For this review, take the finished solid that the model builds, in its own axes (mm). Face numbers are marked on the shaded views. Round coordinates to 2 decimals unless told otherwise and drop trailing zeros. Order: outer loops, then holes, each group sorted by start corner. A loop starts at its lowest first (then second) coordinate and runs counter-clockwise, first axis right, second up. Notation, with made-up numbers: M 0.5,-0.5 L 37.5,-0.5 A31 ccw 37.5,31.5 Z; hole C 67.25,-22 d7. An arc over 180 degrees is marked long. Use a Markdown table: item, result.
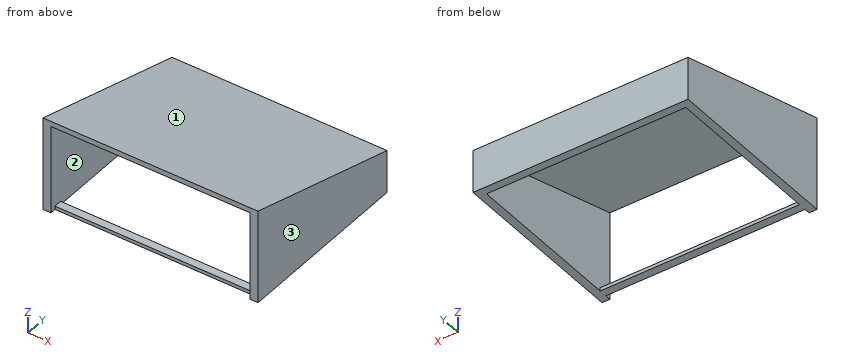
from build123d import *

# Parameters (mm, degrees)
SLOPED_COVER_BLANK_DEPTH                      = 95
SLOPED_COVER_BLANK_DEPTH_BACK                 = 95
OPEN_BOTTOM_AND_FRONT_COVER_CAVITY_DEPTH      = 88
OPEN_BOTTOM_AND_FRONT_COVER_CAVITY_DEPTH_BACK = 88
FRONT_GASKET_COMPRESSION_RAIL_DEPTH           = 95
FRONT_GASKET_COMPRESSION_RAIL_DEPTH_BACK      = 95
FRONT_GASKET_COMPRESSION_RAIL_PROFILE_W       = 3
FRONT_GASKET_COMPRESSION_RAIL_PROFILE_H       = 7


with BuildPart() as part:
    # Sloped Cover Outer Side Profile → Sloped Cover Blank (new, two sides: drawn at the far end of the back side and taken through both)
    with BuildSketch(Plane(origin=(0, 0, 0), x_dir=(0, 0, -1), z_dir=(1, 0, 0)).offset(-SLOPED_COVER_BLANK_DEPTH_BACK)):
        Polygon((-22, 40), (-22, 200), (-60, 200), (-105, 40), align=None)
    extrude(amount=SLOPED_COVER_BLANK_DEPTH + SLOPED_COVER_BLANK_DEPTH_BACK)

    # Open Bottom Cover Cavity Profile → Open Bottom and Front Cover Cavity (cut, two sides: drawn at the far end of the back side and taken through both)
    with BuildSketch(Plane(origin=(0, 0, 0), x_dir=(0, 0, -1), z_dir=(1, 0, 0)).offset(-OPEN_BOTTOM_AND_FRONT_COVER_CAVITY_DEPTH_BACK)):
        Polygon((-18, 38), (-18, 193), (-56, 193), (-101, 38), align=None)
    extrude(amount=OPEN_BOTTOM_AND_FRONT_COVER_CAVITY_DEPTH + OPEN_BOTTOM_AND_FRONT_COVER_CAVITY_DEPTH_BACK, mode=Mode.SUBTRACT)

    # Front Gasket Compression Rail Profile → Front Gasket Compression Rail (add, two sides: drawn at the far end of the back side and taken through both)
    with BuildSketch(Plane(origin=(0, 0, 0), x_dir=(0, 0, -1), z_dir=(1, 0, 0)).offset(-FRONT_GASKET_COMPRESSION_RAIL_DEPTH_BACK)):
        with Locations((-23.5, 48.5)):
            Rectangle(FRONT_GASKET_COMPRESSION_RAIL_PROFILE_W, FRONT_GASKET_COMPRESSION_RAIL_PROFILE_H)
    extrude(amount=FRONT_GASKET_COMPRESSION_RAIL_DEPTH + FRONT_GASKET_COMPRESSION_RAIL_DEPTH_BACK)


solid = part.part
Q1. Clearance check with flat-ended pins moving along their axes: pin 1 (5.5 mm diameter, centred on x = -4.5, y = 48, fed in from +Z); pin 2 (10 mm diameter, centred on x = -8, z = 33.5, fed in from -Y); pin 3 (8 mm diameter, centred on x = -37, y = 84.5, fed in from +Z). State where each tip first meets the part, or that it passes through.
Determined:
| item | result |
|---|---|
| pin 1 | stops at z = 103.52 |
| pin 2 | stops at y = 193 |
| pin 3 | stops at z = 93.61 |
Q2. Wall thickness on line 1 along X through (y, z) = (56.5, 38); line 2 along Y through (x, z) = (-68, 54.5); line 3 along Z through (x, y) = (-8, 48.5): over which ranges is each line inside the solid? List them lowest first. Write a range as [from, to].
Determined:
| item | result |
|---|---|
| line 1 | x = [-95, -88], [88, 95] |
| line 2 | y = [193, 200] |
| line 3 | z = [22, 25], [97.95, 102.61] |
Q3. Add section B-B (z = 52.5). Write out the cut boundary in (x, y).
Determined:
| item | result |
|---|---|
| outline | M -95,40 L -88,40 L -88,193 L 88,193 L 88,40 L 95,40 L 95,200 L -95,200 Z |
Q4. Draft analysis for pull direction X (two halves, no side actions). For the marked faces 1, 2 and 3, state which applies: pulls with the +X half, pulls with the -X half, needs draft (parallel to the pull), parting line crosses it, or undercut.
Determined:
| item | result |
|---|---|
| face 1 | needs draft |
| face 2 | undercut |
| face 3 | pulls with the +X half |
Q5. Add section C-C (y = 68). Write out the cut boundary in (x, z) (3 decimals).
Determined:
| item | result |
|---|---|
| outline | M -95,22 L -88,22 L -88,92.29 L 88,92.29 L 88,22 L 95,22 L 95,97.125 L -95,97.125 Z |
Q6. Add section A-A (x = 16.5). Write out the cut boundary in (y, z), then the cut area to 3 significant figures.
Determined:
| item | result |
|---|---|
| outline | M 40,100.42 L 193,56 L 193,22 L 200,22 L 200,60 L 40,105 Z; M 45,22 L 52,22 L 52,25 L 45,25 Z |
| area | 1,100 mm^2 |
